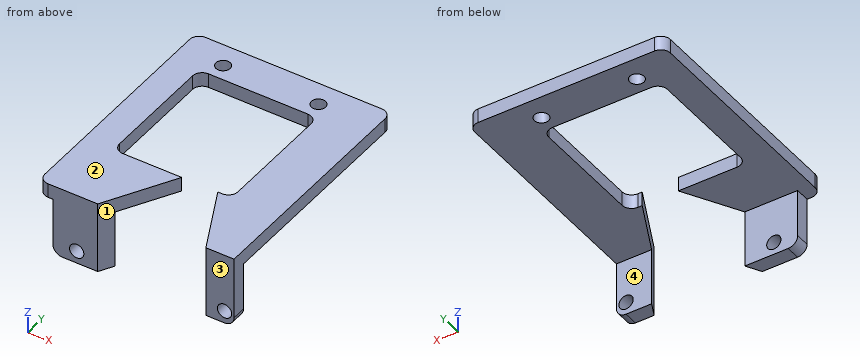
Autodesk Inventor part; units mm, degrees
ref_plane "YZ Plane" through (0, 0, 0) normal (1, 0, 0) x (0, 1, 0)
ref_plane "XZ Plane" through (0, 0, 0) normal (0, 1, 0) x (-1, 0, 0)
ref_plane "XY Plane" through (0, 0, 0) normal (0, 0, 1) x (1, 0, 0)
sketch "Sketch1" plane through (0, 0, 0) normal (0, 0, 1) x (1, 0, 0)
  line L0 (0, 0) -> (53, 0)
  line L1 (53, 0) -> (53, -50)
  line L2 (53, -50) -> (0, -50)
  line L3 (0, -50) -> (0, 0)
  line L4 (41, 0) -> (41, 6.0159) construction
  line L5 (41, 6.0159) -> (41, -25.0024) construction
  circle A0 centre (41, -5) radius 1.5
  line L6 (41, 3.3654) -> (9, 3.3654) construction
  line L7 (9, 3.3654) -> (9, -23.8563) construction
  line L8 (41, -5) -> (7.1054, -5) construction
  circle A1 centre (9, -5) radius 1.5
  line L9 (41, -9) -> (21, -9) construction
  line L10 (21, -9) -> (21, -3) construction
  circle A2 centre (21, -5) radius 1.5
  dimension "d0" = 53
  dimension "d1" = 50
  dimension "d2" = 3
  dimension "d3" = 32
  dimension "d4" = 3
  dimension "d87" = 20
  dimension "d88" = 3
extrude "Extrusion1" add sketch "Sketch1" along normal blind 3 contours L0 L1 L2 L3 | A2
sketch "Sketch2" plane through (0, 0, 3) normal (0, 0, 1) x (1, 0, 0)
  line L0 (53, -50) -> (15, -50)
  line L1 (15, -50) -> (15, -47)
  line L2 (15, -47) -> (53, -47)
  line L3 (53, -47) -> (53, -50)
  dimension "d7" = 38
  dimension "d8" = 3
extrude "Extrusion2" add sketch "Sketch2" against normal blind 15
fillet "Fillet3" radius 2 1 edges at (53, -48.5, -12)
fillet "Fillet6" radius 2 1 edges at (15, -48.5, -12)
sketch "Sketch5" plane through (0, 0, 3) normal (0, 0, 1) x (1, 0, 0)
  line L0 (18.1552, -8.3715) -> (42.9873, -8.3715)
  line L1 (42.9873, -8.3715) -> (42.9873, -35.5989)
  line L2 (42.9873, -35.5989) -> (18.1552, -35.5989)
  line L3 (18.1552, -35.5989) -> (18.1552, -8.3715)
extrude "Extrusion4" cut sketch "Sketch5" against normal through all
fillet "Fillet8" radius 2 1 edges at (18.1552, -8.3715, 1.5)
fillet "Fillet9" radius 2 1 edges at (42.9873, -8.3715, 1.5)
fillet "Fillet10" radius 2 1 edges at (18.1552, -35.5989, 1.5)
fillet "Fillet12" radius 2 1 edges at (42.9873, -35.5989, 1.5)
fillet "Fillet13" radius 2 1 edges at (0, 0, 1.5)
fillet "Fillet14" radius 2 1 edges at (53, 0, 1.5)
sketch "Sketch6" plane through (0, -50, 3) normal (0, -1, 0) x (1, 0, 0)
  line L0 (51, -15) -> (17, -15)
  line L1 (0, 0) -> (53, 0)
  line L2 (53, 0) -> (51, 0) construction
  line L3 (51, 2) -> (51, -15) construction
  line L4 (54, -12.3563) -> (12.4146, -12.3563) construction
  line L5 (51, -7.4819) -> (20, -7.4819) construction
  line L6 (20, -7.4819) -> (20, -11) construction
  circle A0 centre (20, -12.3563) radius 1.5
  circle A1 centre (51, -12.3563) radius 1.5
  dimension "d60" = 31
  dimension "d61" = 3
  dimension "d64" = 3
extrude "Extrusion5" cut sketch "Sketch6" against normal through all contours A0
extrude "Extrusion6" cut sketch "Sketch6" against normal through all contours A1
sketch "Sketch7" plane through (0, 0, 3) normal (0, 0, 1) x (1, 0, 0)
  line L0 (40.9873, -35.5989) -> (20.1552, -35.5989)
  line L1 (0, -50) -> (53, -50)
  line L2 (32.5151, -35.5989) -> (24.407, -50)
  line L3 (40.0869, -35.5989) -> (47.0869, -50)
  point P0 (0, 0)
extrude "Extrusion7" cut sketch "Sketch7" against normal through all
sketch "Sketch8" plane through (0, 0, 3) normal (0, 0, 1) x (1, 0, 0)
  line L0 (0, -50) -> (24.407, -50)
  circle A0 centre (9, -5) radius 1.5
  line L1 (0, 0) -> (12, 0)
  line L2 (12, 0) -> (12, -50)
  line L3 (12, -50) -> (0, -50)
  line L4 (0, -50) -> (0, 0)
extrude "Extrusion8" cut sketch "Sketch8" against normal through all
fillet "Fillet15" radius 2 1 edges at (12, -50, 1.5)
fillet "Fillet16" radius 2 1 edges at (12, 0, 1.5)
hole "Hole4" at (20, -50, -9.3563) direction (0, 1, 0) diameter 3 end through all
hole "Hole5" at (20, -50, -9.3563) direction (0, 1, 0) diameter 3 end through all
extrude "Extrusion9" cut sketch "Sketch1" along normal through all contours A2
properties part number "bart z endstop bracket v4"
The model under review builds one solid part; all positions refer to its coordinate system, in mm. Face numbers are marked on the shaded views. A direction names the side the tool comes from. Give positions to 0.01 mm unless a question says otherwise; leave off trailing zeros. Loops run counter-clockwise (first coordinate to the right, second up) from the corner with the lowest first, then second, coordinate; pieces in that order, holes last. Notation, with made-up numbers: (81.25, 29) -> (117.25, 29) arc R12 ccw to (117.25, 40) -> close; hole circle Ø5 at (5, -29). An arc over 180 degrees is marked (long way). Answer as a JSON object with one key per item and string values. Group by question number.
Q1. Take a section at C-C (y = -5). Write out the cut boundary in (x, z).
Q2. Draft analysis for pull direction X (two halves, no side actions). For the marked faces 1 and 2, state which applies: pulls with the +X half, pulls with the -X half, needs draft (parallel to the pull), parting line crosses it, or undercut.
Q3. Take a section at B-B (z = -6.5). Write out the cut boundary in (x, y).
Q4. Wall thickness on line 1 along Y through (x, z) = (41, 1.95); line 2 along Z through (x, y) = (51, -37.5); line 3 along Z through (x, y) = (20, -47.85): over which ranges is each line inside the solid? List them lowest first.
Q5. Take a section at A-A (y = -20). Write out the cut boundary in (x, z).
Q6. Take a section at D-D (z = 0.75). Write out the cut boundary in (x, y).
Q7. Insertion check: pin 1 (8 mm diameter, centred on x = 37.5, y = -21.5, fed in from +Z); pin 2 (5 mm diameter, centred on x = 51, z = -9.36, fed in from +Y); pin 3 (0.9 mm diameter, centred on x = 32, z = 1.5, fed in from -Y); pin 4 (20.5 mm diameter, centred on x = 26, y = -30, fed in from -Z). Each pin has a flat end and moves straight along its axis. Give the tip position at first contact, or say it passes through.
Q8. Tool access review of the marked faces 3 and 4: name each direction out of +Z, -Z, +X, -X, +Y, -Y from which nothing blocks a thin tool from reaching the whole face with its end or side.
Answer below:
{
 "1": {"outline": "(12, 0) -> (19.5, 0) -> (19.5, 3) -> (12, 3) -> close; (22.5, 0) -> (39.5, 0) -> (39.5, 3) -> (22.5, 3) -> close; (42.5, 0) -> (53, 0) -> (53, 3) -> (42.5, 3) -> close"},
 "2": {"face 1": "undercut", "face 2": "needs draft"},
 "3": {"outline": "(15, -50) -> (24.41, -50) -> (26.1, -47) -> (15, -47) -> close; (45.63, -47) -> (47.09, -50) -> (53, -50) -> (53, -47) -> close"},
 "4": {"line 1": "y = -37.48 to -35.6, -8.37 to -6.5, -3.5 to 0", "line 2": "z = 0 to 3", "line 3": "z = -12 to -10.86, -7.86 to 3"},
 "5": {"outline": "(12, 0) -> (18.16, 0) -> (18.16, 3) -> (12, 3) -> close; (42.99, 0) -> (53, 0) -> (53, 3) -> (42.99, 3) -> close"},
 "6": {"outline": "(12, -48) arc R2 ccw to (14, -50) -> (24.41, -50) -> (32.52, -35.6) -> (20.16, -35.6) arc R2 cw to (18.16, -33.6) -> (18.16, -10.37) arc R2 cw to (20.16, -8.37) -> (40.99, -8.37) arc R2 cw to (42.99, -10.37) -> (42.99, -33.6) arc R2 cw to (40.99, -35.6) -> (40.09, -35.6) -> (47.09, -50) -> (53, -50) -> (53, -2) arc R2 ccw to (51, 0) -> (14, 0) arc R2 ccw to (12, -2) -> close; hole circle Ø3 at (21, -5); hole circle Ø3 at (41, -5)"},
 "7": {"pin 1": "passes through", "pin 2": "stops at y = -47", "pin 3": "stops at y = -37.31", "pin 4": "stops at z = 0"},
 "8": {"face 3": "+Z, -Z, +X, -X, -Y", "face 4": "-Z, +X, -X, +Y"}
}
